Geometry check sheet. Reference: the model listing, model coordinates, mm. A direction names the side the tool comes from. Coordinates: 2 decimals unless noted, no trailing zeros. Write each loop counter-clockwise with the first axis right and the second up, starting at its lowest first coordinate (ties: lowest second). Pieces come first, ordered by that corner, then holes. Notation, with made-up numbers: (26, 5) -> (33, 5) arc R23 cw to (33, 40) -> close; hole circle Ø11 at (49.25, 20). An arc over 180 degrees is marked (long way). One line per question, with ' | ' between items.
```python
from build123d import *

# Parameters (mm, degrees)
SKETCH_1_R          = 25
EXTRUDE_1_DEPTH     = 17
SKETCH_4_R          = 15
CUT_EXTRUDE_1_DEPTH = 3
CUT_EXTRUDE_START   = -3
SKETCH_5_R          = 15
CUT_EXTRUDE_2_DEPTH = 3
CUT_EXTRUDE_3_REACH = 44.052
SKETCH_6_R          = 2.5


with BuildPart() as part:
    # 草图1 → 凸台-拉伸1 (new body)
    with BuildSketch(Plane.XY):
        Circle(SKETCH_1_R)
    extrude(amount=EXTRUDE_1_DEPTH)

    # 扫描1: sweep along a curve in space
    with BuildLine() as sweep_1_path:
        ThreePointArc((25, 0, 17), (17.67766953, 17.67766953, 17), (0, 25, 17))
        ThreePointArc((0, 25, 17), (-17.67766953, 17.67766953, 17), (-25, 0, 17))
        ThreePointArc((-25, 0, 17), (-17.67766953, -17.67766953, 17), (0, -25, 17))
        ThreePointArc((0, -25, 17), (17.67766953, -17.67766953, 17), (25, 0, 17))
    # 草图3 → 扫描1 (sweep)
    with BuildSketch(Plane(origin=(0, 0, 0), x_dir=(1, 0, 0), z_dir=(0, 1, 0))):
        with BuildLine():
            Line((25, -17), (25, 0))
            ThreePointArc((25, 0), (28.038998363, -8.5), (25, -17))
        make_face()
    sweep(path=sweep_1_path.line)

    # 草图4 → 切除-拉伸1 (cut)
    with BuildSketch(Plane(origin=(0, 0, 0), x_dir=(-1, 0, 0), z_dir=(0, 0, -1))):
        Circle(SKETCH_4_R)
    extrude(amount=-CUT_EXTRUDE_1_DEPTH, mode=Mode.SUBTRACT)

    # 草图5 → 切除-拉伸2 (cut)
    with BuildSketch(Plane.XY.offset(17).offset(CUT_EXTRUDE_START)):
        with Locations(Location((0, 0, 0), (0, 0, 180))):
            Circle(SKETCH_5_R)
    extrude(amount=CUT_EXTRUDE_2_DEPTH, mode=Mode.SUBTRACT)

    # 草图6 → 切除-拉伸3 (cut, up to next)
    with BuildSketch(Plane(origin=(0, 0, 3), x_dir=(-1, 0, 0), z_dir=(0, 0, -1)), mode=Mode.PRIVATE) as cut_extrude_3_sk1:
        Circle(SKETCH_6_R)
    cut_extrude_3_tool1 = extrude(cut_extrude_3_sk1.sketch, amount=-CUT_EXTRUDE_3_REACH, mode=Mode.PRIVATE) & part.part
    add(cut_extrude_3_tool1.solids().sort_by_distance((0, 0, 3))[0], mode=Mode.SUBTRACT)


solid = part.part
```
(1) Draft check along X on faces 4 (the face through (11, -11, 0)), 5 (the face through (14.985, 0.66, 1.479)). Enter one of: pulls with the +X half, pulls with the -X half, needs draft (parallel to the pull), parting line crosses it, or undercut.
Answers below:
face 4: needs draft | face 5: undercut
(2) Depth check by flat-ended pin: P1, Ø10, axis at y = 2.5, z = 3, coming from the +X side; P2, Ø2, axis at x = -17, y = 4, coming from the -Z side; P3, Ø15, axis at x = -1.5, y = -2.5, coming from the -Z side; P4, Ø6, axis at y = 11.5, z = 8.5, coming from the +X side. Enter the tip coordinate at first touch or a pass-through.
Answers below:
P1: stops at x = 28 | P2: stops at z = 0 | P3: stops at z = 3 | P4: stops at x = 26.72
(3) Cross-section at A-A (z = 3.75). Record the cut outline in (x, y), plus the area to 3 significant figures.
Answers below:
outline: circle Ø54.34 at (0, 0); hole circle Ø5 at (0, 0) | area: 2,300 mm²
(4) Tool access check on faces 1 (the face through (-8.06, -12.65, 15.48)), 2 (the face through (11, -11, 17)), 3 (the face through (-3, 0, 3)). Record the directions out of +Z, -Z, +X, -X, +Y, -Y that give a thin tool (end or side, any length) a straight path to the whole face; none if there is none.
Answers below:
face 1: +Z | face 2: +Z, +X, -X, +Y, -Y | face 3: -Z
(5) Material ranges on line 1 (Z direction, x = -11, y = 1); line 2 (Y direction, x = 6.5, z = 14.75); line 3 (X direction, y = -10, z = 7), recorded low to high.
Answers below:
line 1: z = 3 to 14 | line 2: y = -25.68 to -13.52, 13.52 to 25.68 | line 3: x = -26.11 to 26.11
(6) Cross-section at B-B (z = 7.75). Record the cut outline in (x, y), plus the area to 3 significant figures.
Answers below:
outline: circle Ø56.04 at (0, 0); hole circle Ø5 at (0, 0) | area: 2,450 mm²
